Can you work these out from the drawing? Everything is in mm from the part's minimum corner. A direction names the side the tool comes from. Round coordinates to 2 decimals unless told otherwise and drop trailing zeros. Order: outer loops, then holes, each group sorted by start corner. A loop starts at its lowest first (then second) coordinate and runs counter-clockwise, first axis right, second up. Notation, with made-up numbers: M -22.5,87.5 L 32.5,87.5 A17 ccw 32.5,98.5 Z; hole C 33.5,51.5 d6. An arc over 180 degrees is marked long. Use one line per item in the form item = value. Start each with the question number.
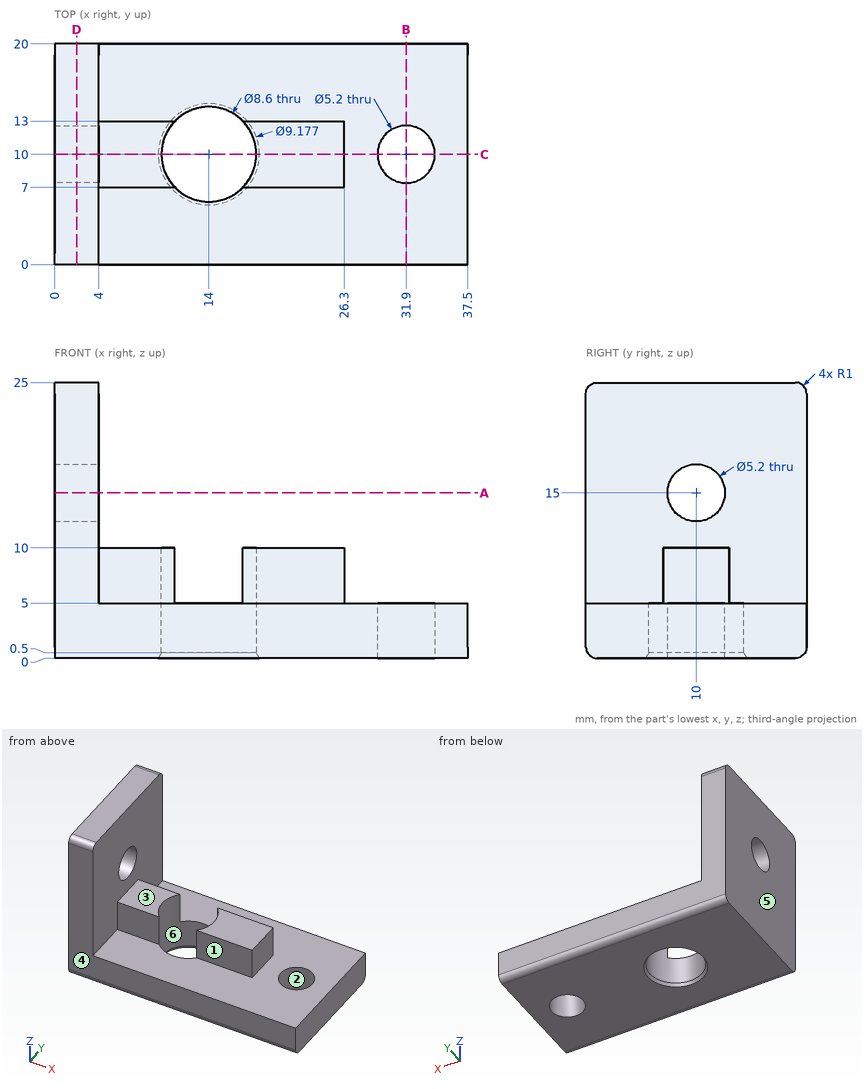
1) If we mould it in two halves opening along Y, with no side actions, what happens to the marked faces 4, 5 and 6? For each: +Y half, -Y half, draft (parallel to the pull), parting line (faces both ways), or undercut.
2) If we section it at D-D on x = 2: Write out the boundary of the cut face in (y, z), then the cut area to 3 significant figures.
3) Will these pins go through, and if not, where does the flat tip stop? pin 1 Ø2.5 at (x, z) = (22, 7.5) entering from +Y; pin 2 Ø4 at (x, y) = (31.9, 10) entering from -Z; pin 3 Ø2.5 at (x, z) = (21, 7.5) entering from -Y; pin 4 Ø8 at (x, y) = (17, 5.5) entering from +Z.
4) If we section it at C-C on y = 10: Write out the boundary of the cut face in (x, z).
5) If we section it at A-A on z = 15: Write out the boundary of the cut face in (x, y).
6) If I drill on line 1 (Z direction, x = 2.75, y = 10); line 2 (X direction, y = 8.5, z = 23); line 3 (Z direction, x = 21.5, y = 2.5), over which ranges is the centre line in solid material (lowest first)?
7) On a 3-axis mill with a long thin cutter (end or side, diameter ignored), from which of +Z, -Z, +X, -X, +Y, -Y can I reach the whole of each face in a straight line? I mean the marked faces 1, 2 and 3. Say none if no direction works.
8) If we section it at B-B on x = 31.9: Write out the boundary of the cut face in (y, z).
Completed:
q1.face_4 = -Y half
q1.face_5 = draft
q1.face_6 = undercut
q2.outline = M 0,1 A1 ccw 1,0 L 19,0 A1 ccw 20,1 L 20,24 A1 ccw 19,25 L 1,25 A1 ccw 0,24 Z; hole C 10,15 d5.2
q2.area = 478 mm²
q3.pin_1 = 13
q3.pin_2 = through
q3.pin_3 = 7
q3.pin_4 = 10
q4.outline = M 0,0 L 9.41,0 L 9.7,0.5 L 9.7,10 L 4,10 L 4,12.4 L 0,12.4 Z; M 0,17.6 L 4,17.6 L 4,25 L 0,25 Z; M 18.3,0.5 L 18.59,0 L 29.3,0 L 29.3,5 L 26.3,5 L 26.3,10 L 18.3,10 Z; M 34.5,0 L 37.5,0 L 37.5,5 L 34.5,5 Z
q5.outline = M 0,0 L 4,0 L 4,7.4 L 0,7.4 Z; M 0,12.6 L 4,12.6 L 4,20 L 0,20 Z
q6.line_1 = 0 to 12.4, 17.6 to 25
q6.line_2 = 0 to 4
q6.line_3 = 0 to 5
q7.face_1 = +Z, +X, -Y
q7.face_2 = +Z, -Z
q7.face_3 = +Z, +X, +Y, -Y
q8.outline = M 0,1 A1 ccw 1,0 L 7.4,0 L 7.4,5 L 0,5 Z; M 12.6,0 L 19,0 A1 ccw 20,1 L 20,5 L 12.6,5 Z
